For this review, take the finished solid that the model builds, in its own axes (mm). A direction names the side the tool comes from. Round coordinates to 2 decimals unless told otherwise and drop trailing zeros. Loops run counter-clockwise (first coordinate to the right, second up) from the corner with the lowest first, then second, coordinate; pieces in that order, holes last.
1) Tool access review of faces 5 (the flat face through (22, 169.84, 0)), 6 (the flat face through (-20.5, 175, 0)), 7 (the flat face through (-11, 159.68, 0)), 8 (the flat face through (0, 20, 0)), 9 (the flat face through (-21, 169.84, 0)): name each direction out of +Z, -Z, +X, -X, +Y, -Y from which nothing blocks a thin tool from reaching the whole face with its end or side.
2) Wall thickness on L1, parallel to X at y = 174.92, z = -7.5; L2, parallel to X at y = 10, z = -8.2; L3, parallel to Y at x = 15, z = -7.5: over which ranges is each line inside the solid? List them lowest first.
3) Take a section at B-B (z = 0). State the section outline as (x, y) points.
4) Take a section at C-C (y = 81.5). State the section outline as (x, z) points, then the cut area to 3 significant figures.
5) Take a section at A-A (x = 0). State the section outline as (y, z) points.
6) Insertion check: pin 1 (6 mm diameter, centred on y = 105.5, z = 0, fed in from +X); pin 2 (1.5 mm diameter, centred on x = -15, y = 174.92, fed in from -Z); pin 3 (1.5 mm diameter, centred on y = 133.5, z = 0.5, fed in from -X); pin 4 (1.5 mm diameter, centred on x = -11, z = -1, fed in from +Y). Each pin has a flat end and moves straight along its axis. Give the tip position at first contact, or say it passes through.
7) Mouldability with a two-part tool opening along Z and no side actions: class faces 1 (the flat face through (14, 172, -3)), 2 (the flat face through (14, 172, 3)), 3 (the flat face through (0, 91, -10)), 4 (the flat face through (9, 0, 2)) as pulls with the +Z half, pulls with the -Z half, needs draft (parallel to the pull), parting line crosses it, or undercut.
Autodesk Inventor part; units mm, degrees
ref_plane "작업 평면1" through (12.5, 0, 0) normal (0, 0, -1) x (-1, 0, 0)
ref_plane "작업 평면2" through (12.5, 0, 0) normal (0, 0, -1) x (-1, 0, 0)
ref_plane "YZ Plane" through (0, 0, 0) normal (1, 0, 0) x (0, 1, 0)
sketch "스케치1" plane through (0, 0, 0) normal (0, 1, 0) x (-1, 0, 0)
  line L0 (-12.5, 10) -> (12.5, 10)
  line L1 (12.5, 10) -> (12.5, -10)
  line L2 (12.5, -10) -> (-12.5, -10)
  line L3 (-12.5, -10) -> (-12.5, 10)
  line L4 (-12.5, 10) -> (12.5, -10) construction
  line L5 (12.5, 10) -> (-12.5, -10) construction
  circle A0 centre (0, 0) radius 8.75
  dimension "d0" = 25
  dimension "d1" = 20
  dimension "d2" = 17.5
extrude "돌출1" add sketch "스케치1" along normal blind 20
sketch "스케치2" plane through (12.5, 0, -10) normal (0, 0, -1) x (-1, 0, 0)
  circle A0 centre (12.5, 10) radius 5
  line L0 (0, 0) -> (25, 0)
  point P0 (12.5, 0)
  point P1 (12.5, 0)
  point P2 (12.5, 0)
  dimension "d5" = 10
  dimension "d6" = 10
extrude "돌출2" cut sketch "스케치2" against normal up to surface (20 mm away)
sketch "스케치3" plane through (0, 20, 0) normal (0, 1, 0) x (1, 0, 0)
  line L0 (12.5, 10) -> (-12.5, 10)
  line L1 (-12.5, 10) -> (-12.5, -10)
  line L2 (-12.5, -10) -> (12.5, -10)
  line L3 (12.5, -10) -> (12.5, 10)
  circle A0 centre (0, 0) radius 8.75
extrude "돌출3" add sketch "스케치3" along normal blind 160 contours L3 L2 L1 L0 | A0
sketch "스케치21" plane through (-12.5, 0, 10) normal (0, 0, 1) x (1, 0, 0)
  line L0 (25, 180) -> (0, 180)
  line L1 (25, 0) -> (25, 180)
  line L2 (0, 180) -> (25, 180)
  line L3 (25, 180) -> (25, 165)
  line L4 (25, 165) -> (0, 165)
  line L5 (0, 165) -> (0, 180)
  point P0 (12.5, 0)
  dimension "d153" = 15
extrude "돌출8" cut sketch "스케치21" against normal blind 0.5
ref_plane "작업 평면1" through (12.5, 0, 0) normal (0, 0, -1) x (-1, 0, 0)
mirror "미러1" about plane through (12.5, 0, 0) normal (0, 0, -1) of "돌출8"
sketch "스케치23" plane through (0, 180, 0) normal (0, 1, 0) x (1, 0, 0)
  circle A0 centre (0, 0) radius 4.5
  line L0 (-2.5981, -4.5) -> (-5.1962, 0)
  line L1 (-5.1962, 0) -> (-2.5981, 4.5)
  line L2 (-2.5981, 4.5) -> (2.5981, 4.5)
  line L3 (2.5981, 4.5) -> (5.1962, 0)
  line L4 (5.1962, 0) -> (2.5981, -4.5)
  line L5 (2.5981, -4.5) -> (-2.5981, -4.5)
  dimension "d162" = 9
extrude "돌출10" cut sketch "스케치23" against normal blind 8
sketch "스케치25" plane through (0, 172, 0) normal (0, 1, 0) x (1, 0, 0)
  line L0 (2.0207, 3.5) -> (4.0415, 0)
  line L1 (4.0415, 0) -> (2.0207, -3.5)
  line L2 (2.0207, -3.5) -> (-2.0207, -3.5)
  line L3 (-2.0207, -3.5) -> (-4.0415, 0)
  line L4 (-4.0415, 0) -> (-2.0207, 3.5)
  line L5 (-2.0207, 3.5) -> (2.0207, 3.5)
  line L6 (-5.1962, 0) -> (-2.5981, 4.5)
  line L7 (2.5981, -4.5) -> (-2.5981, -4.5)
  line L8 (5.1962, 0) -> (2.5981, -4.5)
  line L9 (2.5981, 4.5) -> (5.1962, 0)
  line L10 (-2.5981, 4.5) -> (2.5981, 4.5)
  line L11 (-5.1962, 0) -> (-2.5981, 4.5)
  line L12 (-2.5981, -4.5) -> (-5.1962, 0)
  point P0 (0, 0)
  point P1 (0, 0)
  dimension "d166" = 1
extrude "돌출11" add sketch "스케치25" along normal blind 4.5
sketch "스케치26" plane through (0, 180, 0) normal (0, 1, 0) x (1, 0, 0)
  line L0 (23.5, 10) -> (-23.5, 10)
  line L1 (-23.5, 10) -> (-23.5, -10)
  line L2 (-23.5, -10) -> (23.5, -10)
  line L3 (23.5, -10) -> (23.5, 10)
  line L4 (23.5, 10) -> (-23.5, -10) construction
  line L5 (-23.5, 10) -> (23.5, -10) construction
  line L6 (-9.5, 3) -> (-20.5, 3)
  line L7 (-20.5, 3) -> (-20.5, -3)
  line L8 (-20.5, -3) -> (-9.5, -3)
  line L9 (-9.5, -3) -> (-9.5, 3)
  line L10 (-9.5, 3) -> (-20.5, -3) construction
  line L11 (-20.5, 3) -> (-9.5, -3) construction
  line L12 (-12.5, -9.5) -> (12.5, -9.5)
  line L13 (0, -9.5) -> (0, 10)
  line L14 (-5, 10) -> (5, 10)
  line L15 (23.5, 10) -> (23.5, -10)
  line L16 (9.5, 3) -> (20.5, 3)
  line L17 (20.5, 3) -> (20.5, -3)
  line L18 (20.5, -3) -> (9.5, -3)
  line L19 (9.5, -3) -> (9.5, 3)
  point P0 (0, 0)
  point P1 (-15, 0)
  dimension "d169" = 15
  dimension "d170" = 11
  dimension "d172" = 3
  dimension "d173" = 6
  dimension "d174" = 7
extrude "돌출12" add sketch "스케치26" against normal blind 10.16
sketch "스케치27" plane through (0, 180, 0) normal (0, 1, 0) x (1, 0, 0)
  line L0 (-9.5, 3) -> (-12.5, 3)
  line L1 (-12.5, 3) -> (-12.5, -3)
  line L2 (-12.5, -3) -> (-9.5, -3)
  line L3 (-9.5, -3) -> (-9.5, 3)
  line L4 (-9.5, 3) -> (-12.5, -3) construction
  line L5 (-12.5, 3) -> (-9.5, -3) construction
  line L6 (0, 0) -> (0, 9.5)
  line L7 (12.5, 9.5) -> (-12.5, 9.5)
  line L8 (9.5, 3) -> (12.5, 3)
  line L9 (12.5, 3) -> (12.5, -3)
  line L10 (12.5, -3) -> (9.5, -3)
  line L11 (9.5, -3) -> (9.5, 3)
  line L12 (9.5, 3) -> (12.5, -3) construction
  line L13 (12.5, 3) -> (9.5, -3) construction
  point P0 (-11, 0)
  point P1 (11, 0)
  dimension "d177" = 9.5
  dimension "d178" = 3
  dimension "d179" = 6
extrude "돌출13" cut sketch "스케치27" against normal blind 20.32
sketch "스케치28" plane through (-12.5, 0, 10) normal (0, 0, 1) x (1, 0, 0)
  line L0 (7.5, 87.5) -> (17.5, 87.5)
  line L1 (17.5, 87.5) -> (17.5, 77.5)
  line L2 (17.5, 77.5) -> (7.5, 77.5)
  line L3 (7.5, 77.5) -> (7.5, 87.5)
  line L4 (7.5, 87.5) -> (17.5, 77.5) construction
  line L5 (17.5, 87.5) -> (7.5, 77.5) construction
  line L6 (0, 0) -> (25, 0)
  line L7 (0, 0) -> (0, 165)
  point P0 (12.5, 0)
  point P1 (12.5, 82.5)
  point P2 (12.5, 0)
  point P3 (0, 82.5)
  dimension "d184" = 10
  dimension "d185" = 10
sketch "스케치29" plane through (12.5, 165, -9.5) normal (0, 0, -1) x (-1, 0, 0)
  line L0 (0, 0) -> (25, 0)
  line L1 (25, 4.84) -> (25, 0)
  line L2 (0, 0) -> (0, 4.84)
  line L3 (25, 4.84) -> (0, 4.84)
  point P0 (12.5, -165)
extrude "돌출14" add sketch "스케치29" along normal blind 0.5
ref_plane "작업 평면2" through (12.5, 0, 0) normal (0, 0, -1) x (-1, 0, 0)
mirror "미러2" about plane through (12.5, 0, 0) normal (0, 0, -1) of "돌출14"
sketch "스케치30" plane through (-12.5, 0, 10) normal (0, 0, 1) x (1, 0, 0)
  circle A0 centre (27.5, 174.92) radius 1.25
  line L0 (36, 180) -> (36, 169.84)
  line L1 (0, 0) -> (0, 169.84)
  line L2 (25, 0) -> (25, 169.84)
  line L3 (0, 169.84) -> (25, 169.84)
  line L4 (25, 169.84) -> (12.5, 169.84)
  line L5 (-11, 180) -> (36, 180)
  line L6 (12.5, 180) -> (12.5, 169.84)
  circle A1 centre (-2.5, 174.92) radius 1.25
  point P0 (12.5, 0)
  point P1 (36, 174.92)
  dimension "d186" = 2.5
  dimension "d187" = 8.5
extrude "돌출15" cut sketch "스케치30" against normal up to surface (20 mm away)
equation "\"d34\" = 55deg"
equation "\"d54\" = 55deg"
equation "\"d74\" = 55deg"
equation "\"d94\" = 55deg"
equation "\"d116\" = 55deg"
equation "\"d136\" = 55deg"
properties part number "Tensile_test_bottom_adapter_blocked"
Response:
1. face 5: +Z, -Z, +X, -Y
1. face 6: +Y, -Y
1. face 7: -X, +Y
1. face 8: -Y
1. face 9: +Z, -Z, -X, -Y
2. L1: x = -23.5 to -16.25, -13.75 to 13.75, 16.25 to 23.5
2. L2: x = -12.5 to -5, 5 to 12.5
2. L3: y = 169.84 to 173.67, 176.17 to 180
3. outline: (-23.5, 169.84) - (-20.5, 169.84) - (-20.5, 180) - (-23.5, 180) - close; (-12.5, 0) - (-8.75, 0) - (-8.75, 20) - (8.75, 20) - (8.75, 0) - (12.5, 0) - (12.5, 159.68) - (9.5, 159.68) - (9.5, 180) - (-9.5, 180) - (-9.5, 159.68) - (-12.5, 159.68) - close; (20.5, 169.84) - (23.5, 169.84) - (23.5, 180) - (20.5, 180) - close
4. outline: (-12.5, -10) - (12.5, -10) - (12.5, 10) - (-12.5, 10) - close
4. area: 500 mm2
5. outline: (0, -10) - (5, -10) - (5, -8.75) - (0, -8.75) - close; (0, 8.75) - (5, 8.75) - (5, 10) - (0, 10) - close; (15, -10) - (180, -10) - (180, 10) - (15, 10) - (15, 8.75) - (20, 8.75) - (20, -8.75) - (15, -8.75) - close
6. pin 1: stops at x = 12.5
6. pin 2: passes through
6. pin 3: stops at x = -12.5
6. pin 4: stops at y = 159.68
7. face 1: undercut
7. face 2: undercut
7. face 3: pulls with the -Z half
7. face 4: needs draft
